For this review, take the finished solid that the model builds, in its own axes (mm). Face numbers are marked on the shaded views. A direction names the side the tool comes from. Give positions to 0.01 mm unless a question says otherwise; leave off trailing zeros. Order: outer loops, then holes, each group sorted by start corner. A loop starts at its lowest first (then second) coordinate and runs counter-clockwise, first axis right, second up. Notation, with made-up numbers: (19.5, 79) - (41.5, 79) arc R19 ccw to (41.5, 108) - close; hole circle Ø2 at (-19.5, 75.5). An arc over 180 degrees is marked (long way). Use a Markdown table: item, result. Add a question column.
1) We need section A-A on x = 0. Write out the cut boundary in (y, z), then the cut area to 3 significant figures.
2) Mouldability with a two-part tool opening along Y and no side actions: class the marked faces 1, 2 and 3 as released by +Y, released by -Y, zero draft, split by the parting line, or undercut.
3) Clearance check with flat-ended pins moving along their axes: P1, Ø4, axis at x = -4, z = 6, coming from the -Y side; P2, Ø3, axis at x = -3, z = 3, coming from the +Y side; P3, Ø2, axis at x = -6, z = 3.5, coming from the +Y side. State where each tip first meets the part, or that it passes through.
4) Wall thickness on L1, parallel to X at y = 4, z = 5.75; L2, parallel to Y at x = -8.25, z = 3.25; L3, parallel to X at y = -7, z = 7.75: over which ranges is each line inside the solid? List them lowest first.
5) We need section B-B on x = -4.25. Give the number of separate pieces and of enclosed holes in the cut face, then the cut area to 3 significant figures.
6) Machinability: for the marked faces 4 and 5, which of the approach directions +Z, -Z, +X, -X, +Y, -Y give a long, thin tool a straight path to every point of the face, cutting with its end or side? Answer none if there is none.
```python
from build123d import *

# Parameters (mm, degrees)
SKETCH1_R           = 2.5
BOSS_EXTRUDE2_DEPTH = 10
CUT_EXTRUDE1_REACH  = 18.874
SKETCH2_R           = 2.5


with BuildPart() as part:
    # Sketch1 → Boss-Extrude2 (new body)
    with BuildSketch(Plane.XY):
        with BuildLine():
            add(Edge.make_bspline(
                [(9.610904716, 2.762337877), (8.044691719, 1.282669722), (5.912491895, 1.020999313)],
                knots=[0, 0, 0, 1, 1, 1], degree=2))
            ThreePointArc((9.610904716, 2.762337877), (9.238795325, 3.826834324), (8.749203742, 4.842668053))
            add(Edge.make_bspline(
                [(8.749203742, 4.842668053), (6.595440526, 4.781471609), (4.90271865, 3.458807575)],
                knots=[0, 0, 0, 1, 1, 1], degree=2))
            ThreePointArc((4.90271865, 3.458807575), (4.242640687, 4.242640687), (3.458807575, 4.90271865))
            add(Edge.make_bspline(
                [(4.842668053, 8.749203742), (4.781471609, 6.595440526), (3.458807575, 4.90271865)],
                knots=[0, 0, 0, 1, 1, 1], degree=2))
            ThreePointArc((4.842668053, 8.749203742), (3.826834324, 9.238795325), (2.762337877, 9.610904716))
            add(Edge.make_bspline(
                [(2.762337877, 9.610904716), (1.282669722, 8.044691719), (1.020999313, 5.912491895)],
                knots=[0, 0, 0, 1, 1, 1], degree=2))
            ThreePointArc((1.020999313, 5.912491895), (0, 6), (-1.020999313, 5.912491895))
            add(Edge.make_bspline(
                [(-2.762337877, 9.610904716), (-1.282669722, 8.044691719), (-1.020999313, 5.912491895)],
                knots=[0, 0, 0, 1, 1, 1], degree=2))
            ThreePointArc((-2.762337877, 9.610904716), (-3.826834324, 9.238795325), (-4.842668053, 8.749203742))
            add(Edge.make_bspline(
                [(-4.842668053, 8.749203742), (-4.781471609, 6.595440526), (-3.458807575, 4.90271865)],
                knots=[0, 0, 0, 1, 1, 1], degree=2))
            ThreePointArc((-3.458807575, 4.90271865), (-4.242640687, 4.242640687), (-4.90271865, 3.458807575))
            add(Edge.make_bspline(
                [(-8.749203742, 4.842668053), (-6.595440526, 4.781471609), (-4.90271865, 3.458807575)],
                knots=[0, 0, 0, 1, 1, 1], degree=2))
            ThreePointArc((-8.749203742, 4.842668053), (-9.238795325, 3.826834324), (-9.610904716, 2.762337877))
            add(Edge.make_bspline(
                [(-9.610904716, 2.762337877), (-8.044691719, 1.282669722), (-5.912491895, 1.020999313)],
                knots=[0, 0, 0, 1, 1, 1], degree=2))
            ThreePointArc((-5.912491895, 1.020999313), (-6, 0), (-5.912491895, -1.020999313))
            add(Edge.make_bspline(
                [(-9.610904716, -2.762337877), (-8.044691719, -1.282669722), (-5.912491895, -1.020999313)],
                knots=[0, 0, 0, 1, 1, 1], degree=2))
            ThreePointArc((-9.610904716, -2.762337877), (-9.238795325, -3.826834324), (-8.749203742, -4.842668053))
            add(Edge.make_bspline(
                [(-8.749203742, -4.842668053), (-6.595440526, -4.781471609), (-4.90271865, -3.458807575)],
                knots=[0, 0, 0, 1, 1, 1], degree=2))
            ThreePointArc((-4.90271865, -3.458807575), (-4.242640687, -4.242640687), (-3.458807575, -4.90271865))
            add(Edge.make_bspline(
                [(-4.842668053, -8.749203742), (-4.781471609, -6.595440526), (-3.458807575, -4.90271865)],
                knots=[0, 0, 0, 1, 1, 1], degree=2))
            ThreePointArc((-4.842668053, -8.749203742), (-3.826834324, -9.238795325), (-2.762337877, -9.610904716))
            add(Edge.make_bspline(
                [(-2.762337877, -9.610904716), (-1.282669722, -8.044691719), (-1.020999313, -5.912491895)],
                knots=[0, 0, 0, 1, 1, 1], degree=2))
            ThreePointArc((-1.020999313, -5.912491895), (0, -6), (1.020999313, -5.912491895))
            add(Edge.make_bspline(
                [(2.762337877, -9.610904716), (1.282669722, -8.044691719), (1.020999313, -5.912491895)],
                knots=[0, 0, 0, 1, 1, 1], degree=2))
            ThreePointArc((2.762337877, -9.610904716), (3.826834324, -9.238795325), (4.842668053, -8.749203742))
            add(Edge.make_bspline(
                [(4.842668053, -8.749203742), (4.781471609, -6.595440526), (3.458807575, -4.90271865)],
                knots=[0, 0, 0, 1, 1, 1], degree=2))
            ThreePointArc((3.458807575, -4.90271865), (4.242640687, -4.242640687), (4.90271865, -3.458807575))
            add(Edge.make_bspline(
                [(8.749203742, -4.842668053), (6.595440526, -4.781471609), (4.90271865, -3.458807575)],
                knots=[0, 0, 0, 1, 1, 1], degree=2))
            ThreePointArc((8.749203742, -4.842668053), (9.238795325, -3.826834324), (9.610904716, -2.762337877))
            add(Edge.make_bspline(
                [(9.610904716, -2.762337877), (8.044691719, -1.282669722), (5.912491895, -1.020999313)],
                knots=[0, 0, 0, 1, 1, 1], degree=2))
            ThreePointArc((5.912491895, -1.020999313), (6, 0), (5.912491895, 1.020999313))
        make_face()
        with Locations((0, 0.23341784)):
            Circle(SKETCH1_R, mode=Mode.SUBTRACT)
    extrude(amount=BOSS_EXTRUDE2_DEPTH)

    # Sketch2 → Cut-Extrude1 (cut, up to next)
    with BuildSketch(Plane.XY.offset(10), mode=Mode.PRIVATE) as cut_extrude1_sk1:
        Circle(SKETCH2_R)
    cut_extrude1_tool1 = extrude(cut_extrude1_sk1.sketch, amount=-CUT_EXTRUDE1_REACH, mode=Mode.PRIVATE) & part.part
    add(cut_extrude1_tool1.solids().sort_by_distance((0, 0, 10))[0], mode=Mode.SUBTRACT)


solid = part.part
```
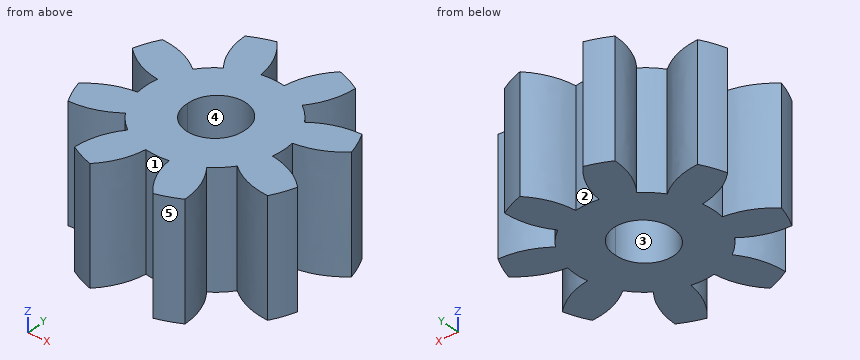
Checked values:
| question | item | result |
|---|---|---|
| 1 | outline | (-6, 0) - (-2.5, 0) - (-2.5, 10) - (-6, 10) - close; (2.73, 0) - (6, 0) - (6, 10) - (2.73, 10) - close |
| 1 | area | 67.7 mm² |
| 2 | face 1 | released by -Y |
| 2 | face 2 | released by +Y |
| 2 | face 3 | undercut |
| 3 | P1 | y = -9.61 |
| 3 | P2 | y = 9.61 |
| 3 | P3 | y = 4.56 |
| 4 | L1 | -9.17 to -5.7, -4.47 to 4.47, 5.7 to 9.17 |
| 4 | L2 | -4.81 to -1.76, 1.76 to 4.81 |
| 4 | L3 | -4.56 to -1.24, 1.24 to 4.56 |
| 5 | separate pieces | 3 |
| 5 | enclosed holes | 0 |
| 5 | area | 142 mm² |
| 6 | face 4 | +Z, -Z |
| 6 | face 5 | +Z, -Z, +X, -Y |
